Print and shaded views of the part. All mm, measured from the part's lowest x, y and z. A direction names the side the tool comes from. Coordinates: 2 decimals unless noted, no trailing zeros. Order: outer loops, then holes, each group sorted by start corner. A loop starts at its lowest first (then second) coordinate and runs counter-clockwise, first axis right, second up. Notation, with made-up numbers: (65, 24.5) -> (82, 24.5) arc R21 ccw to (82, 61.5) -> close; hole circle Ø3 at (-13.5, 10.5). An arc over 180 degrees is marked (long way). Use one line per item in the form item = value. Start each with the question number.
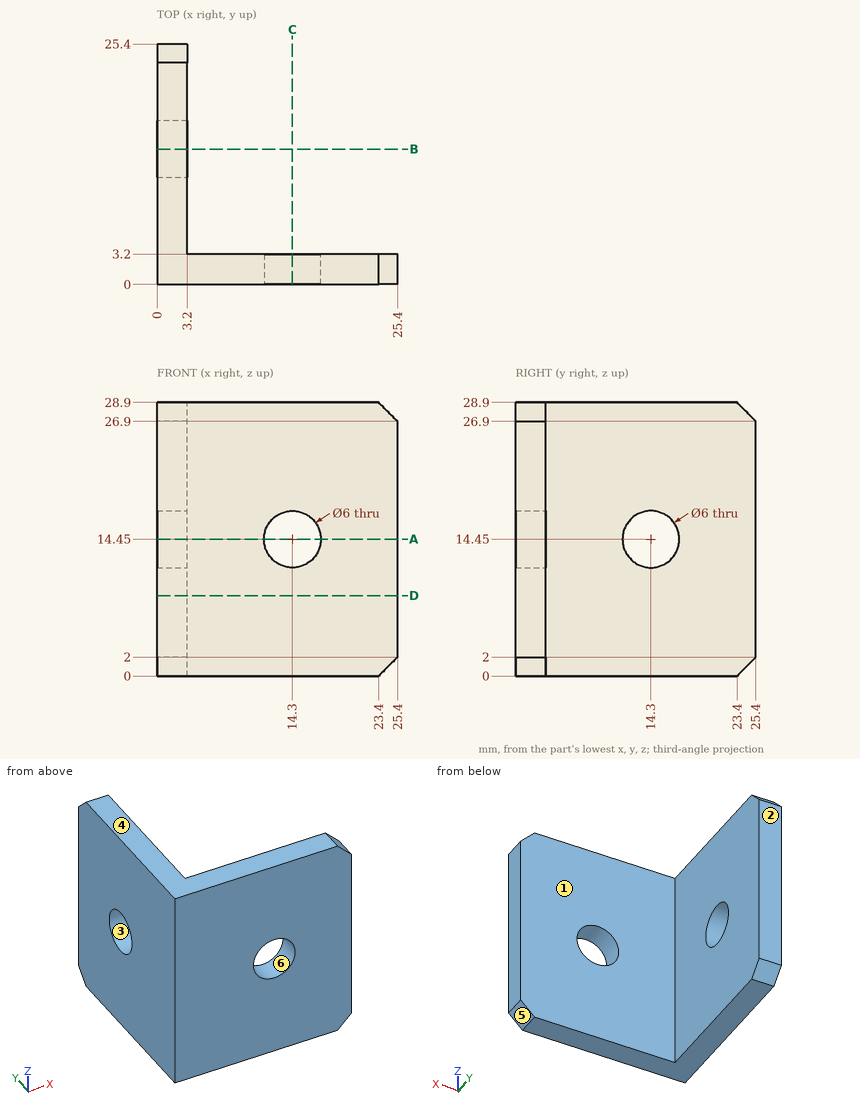
1) Probe L1, parallel to Z at x = 0.7, y = 14.3; L2, parallel to X at y = 4, z = 25.25. List the from-to ranges inside material, lowest first.
2) Drop flat-ended pins along their axis: P1, Ø10, axis at y = 17, z = 21.5, coming from the -X side; P2, Ø1.5, axis at x = 19.5, z = 24.5, coming from the +Y side; P3, Ø2, axis at y = 6, z = 15, coming from the +X side. Give the stop position or say it passes through.
3) Cut at D-D on z = 8.5. Give the cut face in (x, y).
4) Cut at A-A on z = 14.45. Give the cut face in (x, y).
5) Two-plate mould, pull along Z, no slides. Class the marked faces 3, 4, 5 and 6: released by +Z, released by -Z, zero draft, split by the parting line, or undercut.
6) 3-axis set-ups, long thin cutter, end or side, ignore diameter. For the marked faces 1 and 2: which of +Z, -Z, +X, -X, +Y, -Y reach the whole face in a straight line?
7) Cut at B-B on y = 14.3. Give the cut face in (x, z), then the cut area to 3 significant figures.
Values follow:
q1.L1 = 0 to 11.45, 17.45 to 28.9
q1.L2 = 0 to 3.2
q2.P1 = 0
q2.P2 = 3.2
q2.P3 = 3.2
q3.outline = (0, 0) -> (25.4, 0) -> (25.4, 3.2) -> (3.2, 3.2) -> (3.2, 25.4) -> (0, 25.4) -> close
q4.outline = (0, 0) -> (11.3, 0) -> (11.3, 3.2) -> (3.2, 3.2) -> (3.2, 11.3) -> (0, 11.3) -> close; (0, 17.3) -> (3.2, 17.3) -> (3.2, 25.4) -> (0, 25.4) -> close; (17.3, 0) -> (25.4, 0) -> (25.4, 3.2) -> (17.3, 3.2) -> close
q5.face_3 = undercut
q5.face_4 = released by +Z
q5.face_5 = released by -Z
q5.face_6 = undercut
q6.face_1 = +Z, -Z, +X, +Y
q6.face_2 = +Z, -Z, +X, -X, +Y
q7.outline = (0, 0) -> (3.2, 0) -> (3.2, 11.45) -> (0, 11.45) -> close; (0, 17.45) -> (3.2, 17.45) -> (3.2, 28.9) -> (0, 28.9) -> close
q7.area = 73.3 mm^2
